```python
from build123d import *

# Parameters (mm, degrees)
BOSS_EXTRUDE1_DEPTH = 5
SKETCH2_R           = 2
CUT_EXTRUDE1_DEPTH  = 181.346887969


with BuildPart() as part:
    # Sketch1 → Boss-Extrude1 (new body)
    with BuildSketch(Plane(origin=(0, 0, 0), x_dir=(1, 0, 0), z_dir=(0, 1, 0))):
        Polygon((0, 0), (80, 0), (150, -40), (150, -100), (0, -100), align=None)
    extrude(amount=BOSS_EXTRUDE1_DEPTH)

    # Sketch2 → Cut-Extrude1 (cut, through all)
    with BuildSketch(Plane(origin=(0, 5, 0), x_dir=(1, 0, 0), z_dir=(0, 1, 0))):
        with Locations(Location((32, -34, 0), (0, 0, 270))):
            Circle(SKETCH2_R)
        with Locations(Location((40, -34, 0), (0, 0, 270))):
            Circle(SKETCH2_R)
        with Locations(Location((48, -34, 0), (0, 0, 270))):
            Circle(SKETCH2_R)
        with Locations(Location((56, -34, 0), (0, 0, 270))):
            Circle(SKETCH2_R)
        with Locations(Location((64, -34, 0), (0, 0, 270))):
            Circle(SKETCH2_R)
        with Locations(Location((72, -34, 0), (0, 0, 270))):
            Circle(SKETCH2_R)
        with Locations(Location((80, -34, 0), (0, 0, 270))):
            Circle(SKETCH2_R)
        with Locations(Location((88, -34, 0), (0, 0, 270))):
            Circle(SKETCH2_R)
        with Locations(Location((88, -66, 0), (0, 0, 90))):
            Circle(SKETCH2_R)
        with Locations(Location((80, -66, 0), (0, 0, 90))):
            Circle(SKETCH2_R)
        with Locations(Location((72, -66, 0), (0, 0, 90))):
            Circle(SKETCH2_R)
        with Locations(Location((64, -66, 0), (0, 0, 90))):
            Circle(SKETCH2_R)
        with Locations(Location((56, -66, 0), (0, 0, 90))):
            Circle(SKETCH2_R)
        with Locations(Location((48, -66, 0), (0, 0, 90))):
            Circle(SKETCH2_R)
        with Locations(Location((40, -66, 0), (0, 0, 90))):
            Circle(SKETCH2_R)
        with Locations(Location((32, -66, 0), (0, 0, 90))):
            Circle(SKETCH2_R)
        with BuildLine():
            Line((30, -40), (90, -40))
            ThreePointArc((90, -40), (100, -50), (90, -60))
            Line((90, -60), (30, -60))
            ThreePointArc((30, -60), (20, -50), (30, -40))
        make_face()
    extrude(amount=-CUT_EXTRUDE1_DEPTH, mode=Mode.SUBTRACT)


solid = part.part
```
Verification items for the finished model (mm, model axes). A direction names the side the tool comes from. Give positions to 0.01 mm unless a question says otherwise; leave off trailing zeros. Order: outer loops, then holes, each group sorted by start corner. A loop starts at its lowest first (then second) coordinate and runs counter-clockwise, first axis right, second up. Notation, with made-up numbers: (81.25, 84) -> (91.25, 84) arc R19 cw to (91.25, 109) -> close; hole circle Ø2 at (-3.5, 10.5). An arc over 180 degrees is marked (long way). Use a Markdown table: item, result.
1) Section check A-A, the plane x = 48. Record the boundary of the cut face in (y, z).
Results:
| item | result |
|---|---|
| outline | (0, 0) -> (5, 0) -> (5, 32) -> (0, 32) -> close; (0, 36) -> (5, 36) -> (5, 40) -> (0, 40) -> close; (0, 60) -> (5, 60) -> (5, 64) -> (0, 64) -> close; (0, 68) -> (5, 68) -> (5, 100) -> (0, 100) -> close |
2) Mould release check, pull along Z, two halves, no side actions. Record for faces 1 (the cylindrical face through (90, 3, 34)), 2 (the flat face through (150, 2, 70)): pulls with the +Z half, pulls with the -Z half, needs draft (parallel to the pull), parting line crosses it, or undercut.
Results:
| item | result |
|---|---|
| face 1 | undercut |
| face 2 | needs draft |
3) Material ranges on probe 1 along X at (y, z) = (1, 49); probe 2 along X at (y, z) = (2.05, 53.5); probe 3 along Z at (x, y) = (132, 2.25), recorded low to high.
Results:
| item | result |
|---|---|
| probe 1 | 0 to 20.05, 99.95 to 150 |
| probe 2 | 0 to 20.63, 99.37 to 150 |
| probe 3 | 29.71 to 100 |
4) Section check B-B, the plane y = 3.3. Give the number of separate pieces and of enclosed holes in the cut face, then the cut area to 3 significant figures.
Results:
| item | result |
|---|---|
| separate pieces | 1 |
| enclosed holes | 17 |
| area | 11,900 mm² |
5) Section check C-C, the plane x = 96. Record the boundary of the cut face in (y, z), then the cut area to 3 significant figures.
Results:
| item | result |
|---|---|
| outline | (0, 9.14) -> (5, 9.14) -> (5, 42) -> (0, 42) -> close; (0, 58) -> (5, 58) -> (5, 100) -> (0, 100) -> close |
| area | 374 mm² |
6) Tool access check on faces 3 (the flat face through (0, 2, 51)), 4 (the flat face through (60, 3, 40)). Record the directions out of +Z, -Z, +X, -X, +Y, -Y that give a thin tool (end or side, any length) a straight path to the whole face; none if there is none.
Results:
| item | result |
|---|---|
| face 3 | +Z, -Z, -X, +Y, -Y |
| face 4 | +Y, -Y |
7) Depth check by flat-ended pin: pin 1 Ø3 at (x, y) = (71, 3.5) entering from -Z; pin 2 Ø3.5 at (x, z) = (72, 34) entering from +Y. Enter the tip coordinate at first touch or a pass-through.
Results:
| item | result |
|---|---|
| pin 1 | z = 0 |
| pin 2 | through |
